Check sheet for the modelled part. Datum: model origin and axes. Units: mm. A direction names the side the tool comes from. Round coordinates to 2 decimals unless told otherwise and drop trailing zeros. Order: outer loops, then holes, each group sorted by start corner. A loop starts at its lowest first (then second) coordinate and runs counter-clockwise, first axis right, second up. Notation, with made-up numbers: (-36.5, 54) -> (2.5, 54) arc R35 ccw to (2.5, 89) -> close; hole circle Ø2 at (52, -25.75). An arc over 180 degrees is marked (long way). Answer in a Markdown table with one row per item.
```python
from build123d import *

# Parameters (mm, degrees)
BOSS_EXTRUDE4_DEPTH = 60
CUT_EXTRUDE2_DEPTH  = 60
SKETCH8_R           = 2.5
CUT_EXTRUDE3_DEPTH  = 60
CUT_EXTRUDE4_DEPTH  = 26
CUT_EXTRUDE5_DEPTH  = 26
SKETCH11_W          = 44.110265297
SKETCH11_H          = 23.925311971
CUT_EXTRUDE6_DEPTH  = 20
SKETCH12_W          = 40.66810553
SKETCH12_H          = 24.82561344
CUT_EXTRUDE7_DEPTH  = 20
FILLET1_R           = 5
FILLET2_R           = 5
FILLET3_R           = 5
FILLET4_R           = 5
FILLET5_R           = 5
FILLET6_R           = 5
CUT_EXTRUDE8_DEPTH  = 53
CUT_EXTRUDE9_DEPTH  = 40
CUT_EXTRUDE10_DEPTH = 40
CUT_EXTRUDE11_DEPTH = 49
SKETCH17_R          = 1.5
CUT_EXTRUDE12_DEPTH = 20
SKETCH18_R          = 1.5
CUT_EXTRUDE13_DEPTH = 20
SKETCH20_R          = 1.5
CUT_EXTRUDE14_DEPTH = 20
SKETCH21_R          = 1.5
CUT_EXTRUDE15_DEPTH = 20
SKETCH22_R          = 1.5
CUT_EXTRUDE16_DEPTH = 20
SKETCH23_R          = 1.5
CUT_EXTRUDE17_DEPTH = 15
SKETCH24_R          = 1.5
CUT_EXTRUDE18_DEPTH = 15


with BuildPart() as part:
    # Sketch5 → Boss-Extrude4 (new body)
    with BuildSketch(Plane.XY):
        with BuildLine():
            Line((-5.591433469, 0), (-33.737961989, 0))
            ThreePointArc((-33.737961989, 0), (-37.261513388, 1.45252406), (-38.737847513, 4.966165783))
            ThreePointArc((-38.737847513, 4.966165783), (-31.616240623, 53.699065918), (-10.244585549, 98.070962427))
            ThreePointArc((-10.244585549, 98.070962427), (-7.858330599, 99.704279242), (-4.994698694, 99.302347885))
            ThreePointArc((-4.994698694, 99.302347885), (-1.130402236, 95.400824643), (0.061459935, 90.040401592))
            ThreePointArc((0.061459935, 90.040401592), (-0.013962808, 89.477441364), (-0.168362399, 88.93083952))
            ThreePointArc((-0.168362399, 88.93083952), (-7.882068029, 47.204430035), (-1.77951237, 5.212129342))
            ThreePointArc((-1.77951237, 5.212129342), (-2.362771411, 1.638699232), (-5.591433469, 0))
        make_face()
        Polygon((-23.793249775, 26.029552985), (-22.148877555, 31.130017156), (-25.743822989, 35.104317357), (-30.983140641, 33.978153386), (-32.627512861, 28.877689216), (-29.032567427, 24.903389015), align=None, mode=Mode.SUBTRACT)
        Polygon((-19.704548153, 50.537737556), (-20.448711238, 55.006105989), (-24.690513357, 56.595826069), (-28.18815239, 53.717177716), (-27.443989306, 49.248809284), (-23.202187187, 47.659089203), align=None, mode=Mode.SUBTRACT)
        Polygon((-12.020901099, 69.614378519), (-12.60140651, 74.617120781), (-17.224161103, 76.615759479), (-21.266410285, 73.611655915), (-20.685904874, 68.608913653), (-16.063150281, 66.610274955), align=None, mode=Mode.SUBTRACT)
        Polygon((-4.994698694, 87.366252749), (-5.009667304, 90.521352685), (-7.749548306, 92.085939457), (-10.474460698, 90.495426291), (-10.459492087, 87.340326355), (-7.719611085, 85.775739583), align=None, mode=Mode.SUBTRACT)
        Polygon((-12.020901099, 37.637700147), (-12.875266359, 41.812019441), (-16.917515541, 43.159277068), (-20.105399463, 40.332215402), (-19.251034203, 36.157896108), (-15.208785021, 34.810638481), align=None, mode=Mode.SUBTRACT)
        Polygon((-12.020901099, 55.800966029), (-10.82059125, 58.827758896), (-12.841715841, 61.380654151), (-16.063150281, 60.906756539), (-17.263460129, 57.879963671), (-15.242335538, 55.327068416), align=None, mode=Mode.SUBTRACT)
    extrude(amount=BOSS_EXTRUDE4_DEPTH)

    # Sketch7 → Cut-Extrude2 (cut)
    with BuildSketch(Plane.XY.offset(60)):
        with BuildLine():
            Line((-12, 7.5121344), (-7, 7.5121344))
            ThreePointArc((-7, 7.5121344), (-4.4878656, 5), (-7, 2.4878656))
            Line((-7, 2.4878656), (-12, 2.4878656))
            ThreePointArc((-12, 2.4878656), (-14.5121344, 5), (-12, 7.5121344))
        make_face()
    extrude(amount=-CUT_EXTRUDE2_DEPTH, mode=Mode.SUBTRACT)

    # Sketch8 → Cut-Extrude3 (cut)
    with BuildSketch(Plane.XY.offset(60)):
        with Locations((-32.283791832, 6.170765259)):
            Circle(SKETCH8_R)
    extrude(amount=-CUT_EXTRUDE3_DEPTH, mode=Mode.SUBTRACT)

    # Sketch9 → Cut-Extrude4 (cut)
    with BuildSketch(Plane.XY):
        Polygon((0, 0), (-21.41, 0), (-7.180593074, 30.965416872), align=None)
    extrude(amount=CUT_EXTRUDE4_DEPTH, mode=Mode.SUBTRACT)

    # Sketch10 → Cut-Extrude5 (cut)
    with BuildSketch(Plane.XY.offset(60)):
        Polygon((0, 0), (-21.41, 0), (-7.180593074, 30.965416872), align=None)
    extrude(amount=-CUT_EXTRUDE5_DEPTH, mode=Mode.SUBTRACT)

    # Sketch11 → Cut-Extrude6 (cut)
    with BuildSketch(Plane.XY.offset(60)):
        with Locations((-22.055132649, 8.037344015)):
            Rectangle(SKETCH11_W, SKETCH11_H)
    extrude(amount=-CUT_EXTRUDE6_DEPTH, mode=Mode.SUBTRACT)

    # Sketch12 → Cut-Extrude7 (cut)
    with BuildSketch(Plane(origin=(0, 0, 0), x_dir=(-1, 0, 0), z_dir=(0, 0, -1))):
        with Locations((20.334052765, 7.58719328)):
            Rectangle(SKETCH12_W, SKETCH12_H)
    extrude(amount=-CUT_EXTRUDE7_DEPTH, mode=Mode.SUBTRACT)

    # Fillet1
    fillet1_edges = [part.edges().sort_by_distance(p)[0] for p in [
        (-12.219484668, 20, 50),
    ]]
    fillet(fillet1_edges, radius=FILLET1_R)

    # Fillet2
    fillet2_edges = [part.edges().sort_by_distance(p)[0] for p in [
        (-7.180593074, 30.965416872, 47),
    ]]
    fillet(fillet2_edges, radius=FILLET2_R)

    # Fillet3
    fillet3_edges = [part.edges().sort_by_distance(p)[0] for p in [
        (-12.219484668, 20, 10),
    ]]
    fillet(fillet3_edges, radius=FILLET3_R)

    # Fillet4
    fillet4_edges = [part.edges().sort_by_distance(p)[0] for p in [
        (-7.180593074, 30.965416872, 13),
    ]]
    fillet(fillet4_edges, radius=FILLET4_R)

    # Fillet5
    fillet5_edges = [part.edges().sort_by_distance(p)[0] for p in [
        (-38.144186452, 20, 10),
    ]]
    fillet(fillet5_edges, radius=FILLET5_R)

    # Fillet6
    fillet6_edges = [part.edges().sort_by_distance(p)[0] for p in [
        (-38.144186452, 20, 50),
    ]]
    fillet(fillet6_edges, radius=FILLET6_R)

    # Sketch15 → Cut-Extrude8 (cut)
    with BuildSketch(Plane(origin=(0, 0, 0), x_dir=(0, 0, -1), z_dir=(1, 0, 0))):
        Polygon((-60, 20), (-40, 99.809969504), (-60, 99.809969504), align=None)
    extrude(amount=-CUT_EXTRUDE8_DEPTH, mode=Mode.SUBTRACT)

    # Sketch15<2> → Cut-Extrude9 (cut)
    with BuildSketch(Plane(origin=(0, 0, 0), x_dir=(0, 0, -1), z_dir=(1, 0, 0))):
        Polygon((-60, 20), (-40, 99.809969504), (-60, 99.809969504), align=None)
    extrude(amount=CUT_EXTRUDE9_DEPTH, mode=Mode.SUBTRACT)

    # Sketch16 → Cut-Extrude10 (cut)
    with BuildSketch(Plane(origin=(0, 0, 0), x_dir=(0, 0, -1), z_dir=(1, 0, 0))):
        Polygon((0, 20), (0, 99.809969504), (-20, 99.809969504), align=None)
    extrude(amount=-CUT_EXTRUDE10_DEPTH, mode=Mode.SUBTRACT)

    # Sketch16<2> → Cut-Extrude11 (cut)
    with BuildSketch(Plane(origin=(0, 0, 0), x_dir=(0, 0, -1), z_dir=(1, 0, 0))):
        Polygon((0, 20), (0, 99.809969504), (-20, 99.809969504), align=None)
    extrude(amount=CUT_EXTRUDE11_DEPTH, mode=Mode.SUBTRACT)

    # Sketch17 → Cut-Extrude12 (cut)
    with BuildSketch(Plane(origin=(0, 0, 0), x_dir=(0, 0, -1), z_dir=(1, 0, 0))):
        with Locations((-48.227866977, 42.293348251)):
            Circle(SKETCH17_R)
    extrude(amount=-CUT_EXTRUDE12_DEPTH, mode=Mode.SUBTRACT)

    # Sketch18 → Cut-Extrude13 (cut)
    with BuildSketch(Plane(origin=(0, 0, 0), x_dir=(0, 0, -1), z_dir=(1, 0, 0))):
        with Locations((-11.772133023, 42.293348251)):
            Circle(SKETCH18_R)
    extrude(amount=-CUT_EXTRUDE13_DEPTH, mode=Mode.SUBTRACT)

    # Sketch20 → Cut-Extrude14 (cut)
    with BuildSketch(Plane(origin=(0, 0, 0), x_dir=(0, 0, -1), z_dir=(1, 0, 0))):
        with Locations((-30.003246604, 42.293348251)):
            Circle(SKETCH20_R)
    extrude(amount=-CUT_EXTRUDE14_DEPTH, mode=Mode.SUBTRACT)

    # Sketch21 → Cut-Extrude15 (cut)
    with BuildSketch(Plane(origin=(0, 0, 0), x_dir=(0, 0, -1), z_dir=(1, 0, 0))):
        with Locations((-42.714771273, 64.293348251)):
            Circle(SKETCH21_R)
    extrude(amount=-CUT_EXTRUDE15_DEPTH, mode=Mode.SUBTRACT)

    # Sketch22 → Cut-Extrude16 (cut)
    with BuildSketch(Plane(origin=(0, 0, 0), x_dir=(0, 0, -1), z_dir=(1, 0, 0))):
        with Locations((-17.285228727, 64.293348251)):
            Circle(SKETCH22_R)
    extrude(amount=-CUT_EXTRUDE16_DEPTH, mode=Mode.SUBTRACT)

    # Sketch23 → Cut-Extrude17 (cut)
    with BuildSketch(Plane(origin=(0, 0, 0), x_dir=(0, 0, -1), z_dir=(1, 0, 0))):
        with Locations((-37.793709057, 83.93083952)):
            Circle(SKETCH23_R)
    extrude(amount=-CUT_EXTRUDE17_DEPTH, mode=Mode.SUBTRACT)

    # Sketch24 → Cut-Extrude18 (cut)
    with BuildSketch(Plane(origin=(0, 0, 0), x_dir=(0, 0, -1), z_dir=(1, 0, 0))):
        with Locations((-22.206290943, 83.93083952)):
            Circle(SKETCH24_R)
    extrude(amount=-CUT_EXTRUDE18_DEPTH, mode=Mode.SUBTRACT)


solid = part.part
```
(1) Section check C-C on y = 10. Record the boundary of the cut face in (x, z), plus the area to 3 significant figures.
Solutions:
| item | result |
|---|---|
| outline | (-38.69, 20) -> (-16.81, 20) -> (-16.81, 26) -> (-3.2, 26) -> (-3.2, 34) -> (-16.81, 34) -> (-16.81, 40) -> (-38.69, 40) -> close |
| area | 546 mm^2 |
(2) Section check B-B on y = 72. Record the boundary of the cut face in (x, z).
Solutions:
| item | result |
|---|---|
| outline | (-24.79, 13.03) -> (-21.08, 13.03) -> (-21.08, 46.97) -> (-24.79, 46.97) -> close; (-12.3, 13.03) -> (-5.01, 13.03) -> (-5.01, 46.97) -> (-12.3, 46.97) -> close |
(3) Scan lines: probe 1 along Z at (x, y) = (-16.5, 17.5); probe 2 along Y at (x, z) = (-9.5, 33); probe 3 along Y at (x, z) = (-26.5, 41). Record each from-to range of solid material in increasing order. Write a range as from..to.
Solutions:
| item | result |
|---|---|
| probe 1 | 20..40 |
| probe 2 | 0..2.49, 7.51..86.79, 91.06..98.89 |
| probe 3 | 20..25.45, 34.94..48.9, 55.11..68 |
(4) Draft check along Y on faces 1 (the flat face through (-24, 20, 50)), 2 (the flat face through (-28, 10, 20)), 3 (the cylindrical face through (-12.49, 43.78, 48.42)). Enter one of: pulls with the +Y half, pulls with the -Y half, needs draft (parallel to the pull), parting line crosses it, or undercut.
Solutions:
| item | result |
|---|---|
| face 1 | pulls with the -Y half |
| face 2 | needs draft |
| face 3 | undercut |
(5) Section check A-A on x = -9. Give the number of separate pieces and of enclosed holes in the cut face, plus the area to 3 significant figures.
Solutions:
| item | result |
|---|---|
| separate pieces | 3 |
| enclosed holes | 7 |
| area | 2,780 mm^2 |
(6) Depth check by flat-ended pin: pin 1 Ø3.5 at (y, z) = (42, 29.5) entering from +X; pin 2 Ø8 at (y, z) = (65.5, 15) entering from +X; pin 3 Ø5 at (y, z) = (33.5, 15.5) entering from -X; pin 4 Ø3 at (x, z) = (-10, 26.5) entering from -Y. Enter the tip coordinate at first touch or a pass-through.
Solutions:
| item | result |
|---|---|
| pin 1 | x = -7.83 |
| pin 2 | x = -5.52 |
| pin 3 | x = -36.82 |
| pin 4 | y = 0 |
(7) Tool access check on faces 4 (the flat face through (-20, 42, 48)), 5 (the cylindrical face through (-2.332, 1.681, 29.944)), 6 (the flat face through (-12.442, 39.696, 29.642)). Record the directions out of +Z, -Z, +X, -X, +Y, -Y that give a thin tool (end or side, any length) a straight path to the whole face; none if there is none.
Solutions:
| item | result |
|---|---|
| face 4 | +X |
| face 5 | +Z, -Z, +X |
| face 6 | +Z, -Z |
